Geometry check sheet. Reference: the model listing, model coordinates, mm. A direction names the side the tool comes from. Round coordinates to 2 decimals unless told otherwise and drop trailing zeros. Write each loop counter-clockwise with the first axis right and the second up, starting at its lowest first coordinate (ties: lowest second). Pieces come first, ordered by that corner, then holes. Notation, with made-up numbers: M -30,23.5 L 12,23.5 A11 cw 12,31.5 Z; hole C 64,-19 d5. An arc over 180 degrees is marked long. One line per item, written item: value. Start each with the question number.
1. Scan lines: probe 1 along Y at (x, z) = (-68.5, 3.75); probe 2 along Y at (x, z) = (-41.5, 21.5); probe 3 along X at (y, z) = (24.5, 19.5). Record each from-to range of solid material in increasing order. Write a range as [from, to].
2. Release check for a two-part mould opening along Z. For faces 1 (the cylindrical face through (73.609, 37.797, 13.339)), 2 (the cylindrical face through (-0.588, 39.986, 5.004)), 3 (the flat face through (43, 26, 13)) record: pulls with the +Z half, pulls with the -Z half, needs draft (parallel to the pull), parting line crosses it, or undercut.
3. Access from +Z, -Z, +X, -X, +Y, -Y to the whole of each face (thin tool, end or side, straight path). Record for faces 4 (the flat face through (43, 27, 25)), 5 (the cylindrical face through (75.673, 37.226, 25.986)), 6 (the flat face through (34.75, 8, 1)), 7 (the cylindrical face through (76, 13, 5)).
4. Section check C-C (z = 12.75). Count the separate pieces of the cut face and the enclosed holes in it, and give its area (3 significant figures).
5. Section check B-B (x = -28.5). Record the boundary of the cut face in (y, z), and give its area (3 significant figures).
6. Depth check by flat-ended pin: P1, Ø2.5, axis at x = 41, y = 24.5, coming from the +Z side; P2, Ø5.5, axis at x = 43.5, y = 1.5, coming from the +Z side. Enter the tip coordinate at first touch or a pass-through.
7. Section check A-A (y = -21.5). Record the boundary of the cut face in (x, z).
8. Section check D-D (y = 20). Record the boundary of the cut face in (x, z).
from build123d import *

# Parameters (mm, degrees)
F0_W         = 153.5
F0_H         = 82
F1_DEPTH     = 25
F2_W         = 149.5
F2_H         = 78
F3_DEPTH     = 23
F5_DEPTH     = 50
F6_W         = 40
F6_H         = 2
F7_DEPTH     = 23
F8_W         = 69.5
F8_H         = 74
F9_DEPTH     = 2.001
F12_DEPTH    = 25
F14_W        = 2
F14_H        = 26
F14_H_2      = 2
F15_DEPTH    = 23
F17_DEPTH    = 27.001
F19_DEPTH    = 82.001
F20_R        = 2
F21_DEPTH    = 2
F22_T1_DEPTH = 23
F22_T3_DEPTH = 17
F23_R        = 1


# Not quite as in the source:
# - a fillet or chamfer that OpenCascade refuses, or shapes differently, is made with other operations: its cross-section is extruded or revolved along the edge and cut away or added


with BuildPart() as f1:
    # F0 (on Top) → F1 (new body)
    with BuildSketch(Plane.XY):
        Rectangle(F0_W, F0_H)
    extrude(amount=F1_DEPTH)

    # F2 (on face) → F3 (cut)
    with BuildSketch(Plane.XY.offset(25)):
        Rectangle(F2_W, F2_H)
    extrude(amount=-F3_DEPTH, mode=Mode.SUBTRACT)

    # F4 (on face) → F5 (join)
    with BuildSketch(Plane.XZ.offset(-39)):
        Polygon((-34.75, 2), (-74.75, 25), (-74.75, 2), align=None)
    extrude(amount=F5_DEPTH)

    # F6 (on face) → F7 (join)
    with BuildSketch(Plane.XY.offset(2)):
        with Locations((-54.75, -12)):
            Rectangle(F6_W, F6_H)
    extrude(amount=F7_DEPTH)

    # F8 (on face) → F9 (cut, through all)
    with BuildSketch(Plane.XY.offset(2)):
        Rectangle(F8_W, F8_H)
    extrude(amount=-F9_DEPTH, mode=Mode.SUBTRACT)

    # F11 (on face) → F12 (join)
    with BuildSketch(Plane.XY.offset(25)):
        Polygon((-74.75, 39), (-74.75, 30.4142603609), (-34.75, 37), (-34.75, 39), align=None)
        Polygon((-74.75, -11), (-35.1230073053, -11), (-35.1229473745, -10.9961439342), (-74.75, -3.6334587345), align=None)
    extrude(amount=-F12_DEPTH)

    # F14 (on face) → F15 (join)
    with BuildSketch(Plane.XY.offset(2)):
        Polygon((36.75, 26), (49.75, 26), (51.75, 26), (51.75, 28), (34.75, 28), (34.75, 26), align=None)
        with Locations((50.75, 13)):
            Rectangle(F14_W, F14_H)
        Polygon((51.75, 0), (49.75, 0), (36.75, 0), (34.75, 0), (34.75, -2), (51.75, -2), align=None)
        with Locations((35.75, 25)):
            Rectangle(F14_W, F14_H_2)
        with Locations((35.75, 1)):
            Rectangle(F14_W, F14_H_2)
    extrude(amount=F15_DEPTH)

    # F16 (on face) → F17 (cut, through all)
    with BuildSketch(Plane(origin=(49.75, 0, 0), x_dir=(0, -1, 0), z_dir=(-1, 0, 0))):
        with BuildLine():
            Line((-3, 25), (-23, 25))
            Line((-23, 25), (-23, 15))
            ThreePointArc((-23, 15), (-13.0980438814, 4.9995097688), (-3, 14.8019609728))
            Line((-3, 14.8019609728), (-3, 25))
        make_face()
    extrude(amount=-F17_DEPTH, mode=Mode.SUBTRACT)

    # F18 (on face) → F19 (cut, through all)
    with BuildSketch(Plane.XZ.offset(41)):
        with BuildLine():
            Line((34.75, 25), (-34.75, 25))
            ThreePointArc((-34.75, 25), (0, 5), (34.75, 25))
        make_face()
    extrude(amount=-F19_DEPTH, mode=Mode.SUBTRACT)

    # F20 (on face) → F21 (join)
    with BuildSketch(Plane.XY.offset(25)):
        with Locations((-74.75, 39)):
            Circle(F20_R)
        with Locations((74.75, 39)):
            Circle(F20_R)
        with Locations((-74.75, -39)):
            Circle(F20_R)
        with Locations((74.75, -39)):
            Circle(F20_R)
    extrude(amount=F21_DEPTH)

    # F22: fillet of radius 4 on 5 edges, made by hand

    # F22_s2 → F22_t1 (join)
    with BuildSketch(Plane.XY.offset(2)):
        with BuildLine():
            ThreePointArc((-70.75, -39), (-73.5784271247, -37.8284271247), (-74.75, -35))
            Line((-74.75, -35), (-74.75, -39))
            Line((-74.75, -39), (-70.75, -39))
        make_face()
        with BuildLine():
            ThreePointArc((74.75, 35), (73.5784271247, 37.8284271247), (70.75, 39))
            Line((70.75, 39), (74.75, 39))
            Line((74.75, 39), (74.75, 35))
        make_face()
        with BuildLine():
            ThreePointArc((70.75, -39), (73.5784271247, -37.8284271247), (74.75, -35))
            Line((74.75, -35), (74.75, -39))
            Line((74.75, -39), (70.75, -39))
        make_face()
    extrude(amount=F22_T1_DEPTH)

    # F22_s4 → F22_t3 (join)
    with BuildSketch(Plane.YZ.offset(34.75)):
        with BuildLine():
            ThreePointArc((-6, 2), (-3.1715728753, 3.1715728753), (-2, 6))
            Line((-2, 6), (-2, 2))
            Line((-2, 2), (-6, 2))
        make_face()
        with BuildLine():
            ThreePointArc((32, 2), (29.1715728753, 3.1715728753), (28, 6))
            Line((28, 6), (28, 2))
            Line((28, 2), (32, 2))
        make_face()
    extrude(amount=F22_T3_DEPTH)

    # F23
    f23_edges = [f1.edges().sort_by_distance(p)[0] for p in [
        (76.75, -41, 12.5),
        (-76.75, -41, 12.5),
        (-76.75, 41, 12.5),
        (76.75, 41, 12.5),
    ]]
    fillet(f23_edges, radius=F23_R)


solid = f1.part
Result sheet:
1. probe 1: y = [-41, -39], [-13, 41]
1. probe 2: y = [-41, -39], [-13, -9.81], [35.89, 41]
1. probe 3: x = [-76.75, -65.18], [34.75, 36.75], [49.75, 51.75], [74.75, 76.75]
2. face 1: undercut
2. face 2: pulls with the +Z half
2. face 3: needs draft
3. face 4: +Z, +X, -X, +Y, -Y
3. face 5: +Z
3. face 6: +Z, -Z
3. face 7: +Z, +X
4. separate pieces: 5
4. enclosed holes: 0
4. area: 2,040 mm2
5. outline: M -41,0 L -37,0 L -37,2 L -39,2 L -39,16.85 L -41,16.85 Z; M 37,0 L 41,0 L 41,16.85 L 39,16.85 L 39,2 L 37,2 Z
5. area: 75.4 mm2
6. P1: stops at z = 2
6. P2: stops at z = 25
7. outline: M -76.75,0 L -34.75,0 L -34.75,2 L -74.75,2 L -74.75,25 L -76.75,25 Z; M 34.75,0 L 76.75,0 L 76.75,25 L 74.75,25 L 74.75,2 L 34.75,2 Z
8. outline: M -76.75,0 L -34.75,0 L -34.75,2 L -74.75,25 L -76.75,25 Z; M 34.75,0 L 76.75,0 L 76.75,7.86 L 74.75,7.86 L 74.75,2 L 51.75,2 L 51.75,7.86 L 49.75,7.86 L 49.75,2 L 34.75,2 Z
